Answer from the drawing. Dimensions are ordinates in mm from the lowest x, y and z of the part. Coordinates: 2 decimals unless noted, no trailing zeros. Write each loop counter-clockwise with the first axis right and the second up, starting at its lowest first coordinate (ties: lowest second). Pieces come first, ordered by that corner, then holes.
1) The part is cut by section A-A (y = 138.5). Determine the outline of the cut face in (x, z), then the cut area to 3 significant figures.
2) Determine the mould class of the marked faces 1, 2 and 3 for opening direction X: +X half, -X half, draft (parallel to the pull), parting line (faces both ways), or undercut.
3) Find the intervals of material crossed by line 1 (X direction, y = 23, z = 97); line 2 (Z direction, x = 89, y = 186); line 3 (X direction, y = 123.5, z = 7), in increasing order.
4) Each of these flat-tipped pins is pushed along its axis until it touches: pin 1 Ø12 at (x, y) = (26, 71) entering from -Z; pin 2 Ø1.5 at (x, y) = (84.5, 41.5) entering from +Z; pin 3 Ø1 at (y, z) = (78, 14) entering from +X; pin 4 Ø1.5 at (y, z) = (103.5, 11.5) entering from -X (3 decimals). Where does it stop, or does it pass through?
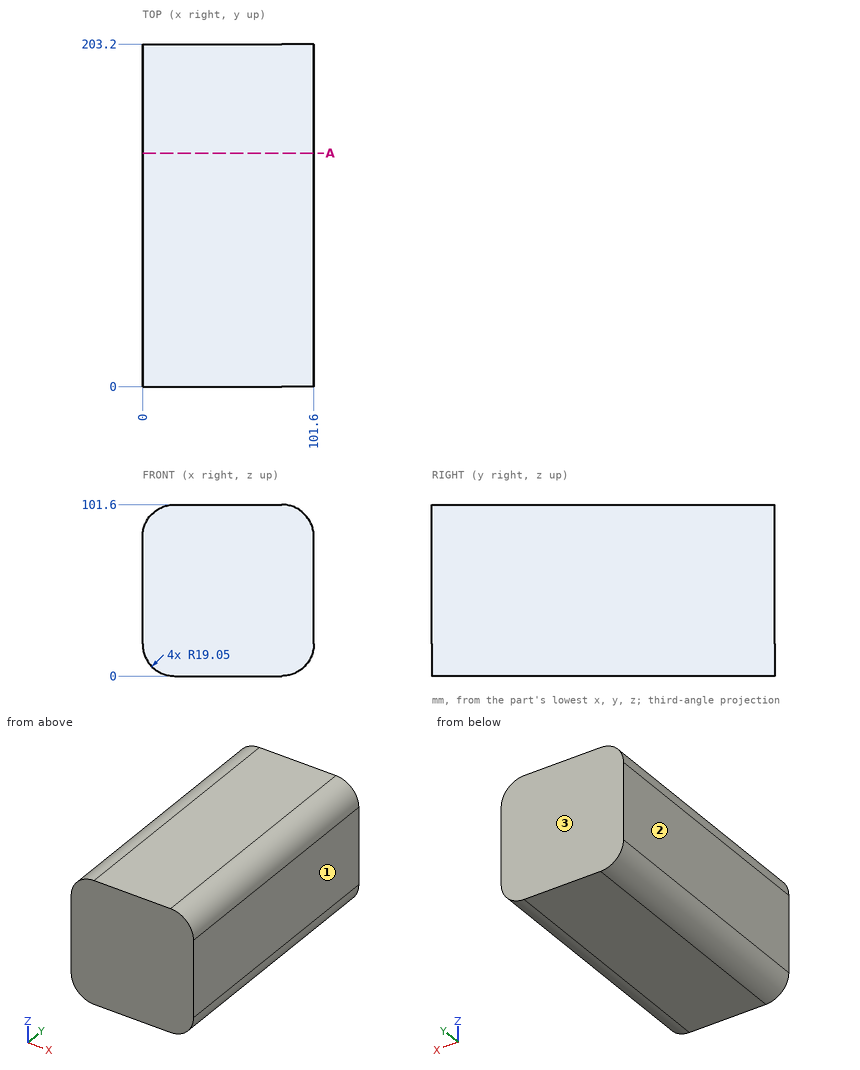
Reported:
1. outline: (0, 19.05) arc R19.05 ccw to (19.05, 0) - (82.55, 0) arc R19.05 ccw to (101.6, 19.05) - (101.6, 82.55) arc R19.05 ccw to (82.55, 101.6) - (19.05, 101.6) arc R19.05 ccw to (0, 82.55) - close
1. area: 10,000 mm2
2. face 1: +X half
2. face 2: -X half
2. face 3: draft
3. line 1: x = 6.64 to 94.96
3. line 2: z = 1.13 to 100.47
3. line 3: x = 4.3 to 97.3
4. pin 1: stops at z = 0
4. pin 2: stops at z = 101.56
4. pin 3: stops at x = 101.05
4. pin 4: stops at x = 1.255
